Part print with two shaded views. Sizes in mm from the minimum x, y, z corner. A direction names the side the tool comes from. Coordinates: 2 decimals unless noted, no trailing zeros. Loops run counter-clockwise (first coordinate to the right, second up) from the corner with the lowest first, then second, coordinate; pieces in that order, holes last.
Item 1: Cut at B-B (x = 17). List the corners of the cut face in (y, z), and give its area (3 significant figures).
Item 2: Cut at C-C (z = 4.75). List the corners of the cut face in (x, y), and give its area (3 significant figures).
Item 3: Cut at D-D (x = 6.25). List the corners of the cut face in (y, z), and give its area (3 significant figures).
Item 4: Drill centre lines: line 1 along Y through (x, z) = (17, 2.75); line 2 along Y through (x, z) = (10.75, 3); line 3 along X through (y, z) = (23, 5.25). Where is each one in solid material? Low to high.
Item 5: 3-axis set-ups, long thin cutter, end or side, ignore diameter. For the marked faces 1 and 2: which of +Z, -Z, +X, -X, +Y, -Y reach the whole face in a straight line?
Item 6: Flat gauge pin, fed straight in: pin 1 (1.5 mm diameter, centred on y = 23.5, z = 3.5, fed in from -X). Where does the tip first touch, or does it go through?
Item 7: Cut at A-A (y = 8). List the corners of the cut face in (x, z), and give its area (3 significant figures).
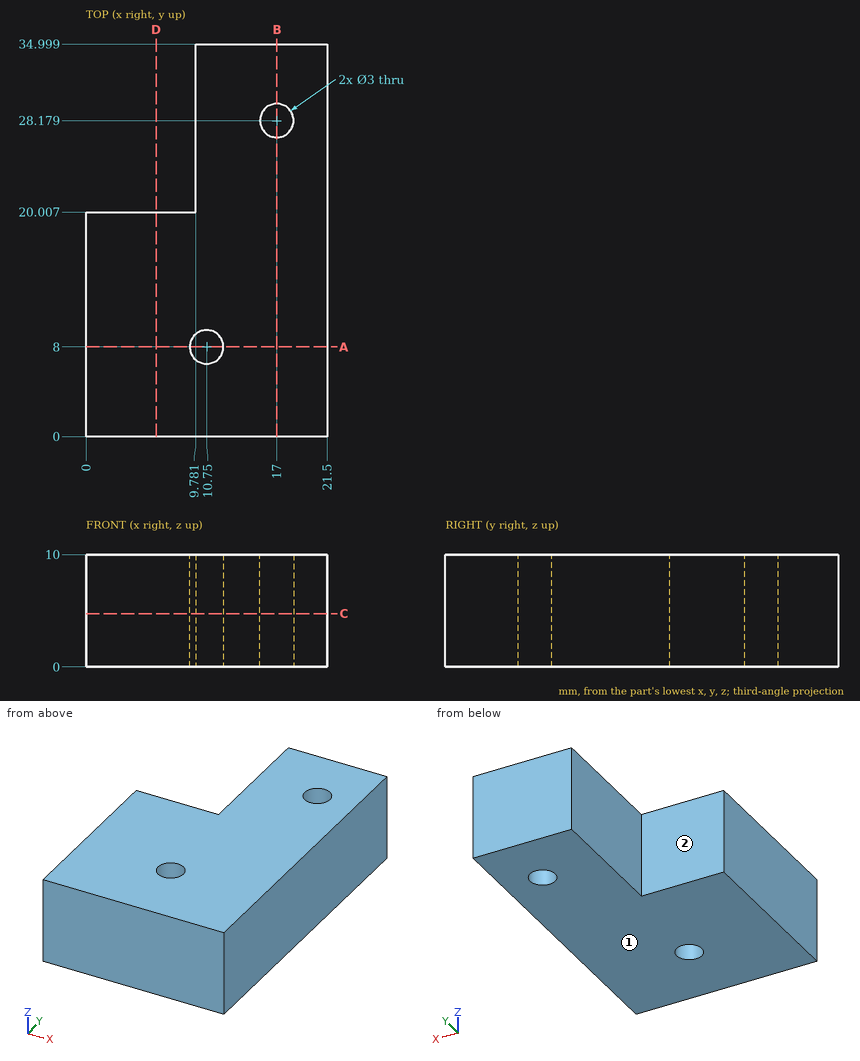
Filled sheet:
1. outline: (0, 0) - (26.68, 0) - (26.68, 10) - (0, 10) - close; (29.68, 0) - (35, 0) - (35, 10) - (29.68, 10) - close
1. area: 320 mm2
2. outline: (0, 0) - (21.5, 0) - (21.5, 35) - (9.78, 35) - (9.78, 20.01) - (0, 20.01) - close; hole circle Ø3 at (10.75, 8); hole circle Ø3 at (17, 28.18)
2. area: 592 mm2
3. outline: (0, 0) - (20.01, 0) - (20.01, 10) - (0, 10) - close
3. area: 200 mm2
4. line 1: y = 0 to 26.68, 29.68 to 35
4. line 2: y = 0 to 6.5, 9.5 to 35
4. line 3: x = 9.78 to 21.5
5. face 1: -Z, +X, -X, +Y, -Y
5. face 2: +Z, -Z, -X, +Y
6. pin 1: stops at x = 9.78
7. outline: (0, 0) - (9.25, 0) - (9.25, 10) - (0, 10) - close; (12.25, 0) - (21.5, 0) - (21.5, 10) - (12.25, 10) - close
7. area: 185 mm2
